Input: part model. Units: mm. Frame: model coordinates. A direction names the side the tool comes from. Give positions to 0.01 mm unless a question says otherwise; leave off trailing zeros. Loops run counter-clockwise (first coordinate to the right, second up) from the corner with the lowest first, then second, coordinate; pieces in that order, holes last. Notation, with made-up numbers: (69.5, -14) -> (90.5, -14) arc R22 ccw to (90.5, 2) -> close; hole circle Ø3 at (-9, 38.5). An arc over 180 degrees is marked (long way). Answer as a JSON object with one key per item and string values.
Autodesk Inventor part; units mm, degrees
ref_plane "YZ Plane" through (0, 0, 0) normal (1, 0, 0) x (0, 1, 0)
ref_plane "XZ Plane" through (0, 0, 0) normal (0, 1, 0) x (-1, 0, 0)
ref_plane "XY Plane" through (0, 0, 0) normal (0, 0, 1) x (1, 0, 0)
sketch "Sketch1" plane through (0, 0, 0) normal (0, 1, 0) x (-1, 0, 0)
  line L0 (0, 0) -> (-58.801, 0)
  line L1 (-58.801, 0) -> (-58.801, 41.275)
  line L2 (-58.801, 41.275) -> (0, 41.275)
  line L3 (0, 41.275) -> (0, 0)
  dimension "d0" = 41.275
  dimension "d1" = 58.801
extrude "Extrusion1" add sketch "Sketch1" against normal blind 2.9972
sketch "Sketch2" plane through (0, 0, 0) normal (0, 1, 0) x (1, 0, 0)
  line L0 (0, -41.275) -> (0, 0)
  line L1 (58.801, -41.275) -> (0, -41.275)
  line L2 (22.4155, -8.5725) -> (36.3855, -8.5725)
  line L3 (36.3855, -8.5725) -> (36.3855, -17.4625)
  line L4 (36.3855, -17.4625) -> (22.4155, -17.4625)
  line L5 (22.4155, -17.4625) -> (22.4155, -8.5725)
  point P0 (29.4005, -13.0175)
  dimension "d7" = 8.89
  dimension "d17" = 13.97
  dimension "d22" = 6.985
  dimension "d23" = 4.445
  dimension "d24" = 29.4005
  dimension "d26" = 28.2575
extrude "Extrusion2" cut sketch "Sketch2" against normal blind 2.9972
fillet "Fillet1" radius 1.5875 4 edges at (22.4155, -1.4986, 8.5725) (22.4155, -1.4986, 17.4625) (36.3855, -1.4986, 17.4625) (36.3855, -1.4986, 8.5725)
properties part number "Lidar Sensor Case 4 v2"
Q1. Draft query along X for faces 3 (the flat face through (58.801, -1, 20)), 4 (the cylindrical face through (35.908, -1.52, 9.025)), 5 (the flat face through (30, -2.997, 21)). Return one class per face: +X half, -X half, draft (parallel to the pull), parting line (faces both ways), or undercut.
Evaluation:
{"face 3": "+X half", "face 4": "undercut", "face 5": "draft"}
Q2. Ray query, line 1 along Z through (x, y) = (32.5, -0.6) (1 decimal); line 2 along Z through (x, y) = (23, -0.7) (1 decimal). Return the intervals inside material, ascending.
Evaluation:
{"line 1": "z = 0 to 8.6, 17.5 to 41.3", "line 2": "z = 0 to 8.9, 17.1 to 41.3"}
Q3. Section B-B, the plane x = 28. Return the cut outline in (y, z) (1 decimal), then the cut area to 3 significant figures.
Evaluation:
{"outline": "(-3, 0) -> (0, 0) -> (0, 8.6) -> (-3, 8.6) -> close; (-3, 17.5) -> (0, 17.5) -> (0, 41.3) -> (-3, 41.3) -> close", "area": "97.1 mm2"}
Q4. Access query for faces 1 (the flat face through (22.416, -1, 13)), 2 (the flat face through (30, 0, 21)). Directions: +Z, -Z, +X, -X, +Y, -Y. A direction counts if a zero-diameter tool reaches every point of the face in a straight line with its end or side. Return the directions, or none.
Evaluation:
{"face 1": "+Y, -Y", "face 2": "+Z, -Z, +X, -X, +Y"}
Q5. Pin query (flat end, axial travel): pin 1 (1.5 mm diameter, centred on x = 29, y = -2, fed in from -Z). Return the tip coordinate at first contact, or that it passes through.
Evaluation:
{"pin 1": "stops at z = 0"}
Q6. Section C-C, the plane y = -1.5. Return the cut outline in (x, z) (1 decimal).
Evaluation:
{"outline": "(0, 0) -> (58.8, 0) -> (58.8, 41.3) -> (0, 41.3) -> close; hole (22.4, 10.2) arc R1.6 ccw to (24, 8.6) -> (34.8, 8.6) arc R1.6 ccw to (36.4, 10.2) -> (36.4, 15.9) arc R1.6 ccw to (34.8, 17.5) -> (24, 17.5) arc R1.6 ccw to (22.4, 15.9) -> close"}
Q7. Section A-A, the plane z = 11. Return the cut outline in (x, y).
Evaluation:
{"outline": "(0, -3) -> (22.42, -3) -> (22.42, 0) -> (0, 0) -> close; (36.39, -3) -> (58.8, -3) -> (58.8, 0) -> (36.39, 0) -> close"}
